```python
from build123d import *

# Parameters (mm, degrees)
EXTRUDE1_DEPTH = 12.7
EXTRUDE2_DEPTH = 216.9
SKETCH8_R      = 9.07761974
EXTRUDE3_DEPTH = 216.9


with BuildPart() as part:
    # Sketch1 → Extrude1 (new body)
    with BuildSketch(Plane(origin=(0, 0, 0), x_dir=(1, 0, 0), z_dir=(0, 1, 0))):
        with BuildLine():
            Line((-131.982271537, 76.2), (-21.997045256, 12.7))
            ThreePointArc((-21.997045256, 12.7), (0, 25.4), (21.997045256, 12.7))
            Line((21.997045256, 12.7), (131.982271537, 76.2))
            ThreePointArc((131.982271537, 76.2), (0, -152.4), (-131.982271537, 76.2))
        make_face()
    extrude(amount=EXTRUDE1_DEPTH)

    # Sketch2 → Extrude2 (cut, through all)
    with BuildSketch(Plane(origin=(0, 12.7, 0), x_dir=(1, 0, 0), z_dir=(0, 1, 0))):
        with BuildLine():
            Line((-122.312523376, 34.185473895), (-25.376324988, -1.096416941))
            ThreePointArc((-25.376324988, -1.096416941), (-20.043874739, -15.601380882), (-7.29146874, -24.33093676))
            Line((-7.29146874, -24.33093676), (-24.958114169, -124.523461794))
            ThreePointArc((-24.958114169, -124.523461794), (-108.255677623, -66.405634267), (-122.312523376, 34.185473895))
        make_face()
        with BuildLine():
            Line((25.376324988, -1.096416941), (122.312523376, 34.185473895))
            ThreePointArc((122.312523376, 34.185473895), (108.43851372, -66.106646732), (25.644983679, -124.38382054))
            Line((25.644983679, -124.38382054), (7.965532589, -24.118670995))
            ThreePointArc((7.965532589, -24.118670995), (20.258971151, -15.321034165), (25.376324988, -1.096416941))
        make_face()
    extrude(amount=-EXTRUDE2_DEPTH, mode=Mode.SUBTRACT)

    # Sketch8 → Extrude3 (cut, through all)
    with BuildSketch(Plane.XZ):
        with Locations(Location((0, 0, 0), (0, 0, 270))):
            Circle(SKETCH8_R)
    extrude(amount=-EXTRUDE3_DEPTH, mode=Mode.SUBTRACT)


solid = part.part
```
The model under review builds one solid part; all positions refer to its coordinate system, in mm. A direction names the side the tool comes from. Coordinates: 2 decimals unless noted, no trailing zeros. Order: outer loops, then holes, each group sorted by start corner. A loop starts at its lowest first (then second) coordinate and runs counter-clockwise, first axis right, second up. Notation, with made-up numbers: M 86,30.5 L 130,30.5 A17 cw 130,59.5 Z; hole C 42.25,12 d10. An arc over 180 degrees is marked long. One line per question, with ' | ' between items.
(1) Add section A-A, the plane x = 0. Write out the cut boundary in (y, z).
Geometry results:
outline: M 0,-25.4 L 12.7,-25.4 L 12.7,-9.08 L 0,-9.08 Z; M 0,9.08 L 12.7,9.08 L 12.7,152.4 L 0,152.4 Z
(2) Insertion check: pin 1 (4 mm diameter, centred on x = 80.5, y = 2, fed in from +Z); pin 2 (6 mm diameter, centred on y = 5, z = -9, fed in from +X); pin 3 (10 mm diameter, centred on x = -110.5, z = -33.5, fed in from -Y); pin 4 (1 mm diameter, centred on x = 93.5, y = 11, fed in from +Z). Each pin has a flat end and moves straight along its axis. Give the tip position at first contact, or say it passes through.
Geometry results:
pin 1: stops at z = 130.63 | pin 2: stops at x = 152.28 | pin 3: stops at y = 0 | pin 4: stops at z = 120.73
(3) Add section B-B, the plane y = 9.25. Write out the cut boundary in (x, z).
Geometry results:
outline: M -131.98,-76.2 L -22,-12.7 A25.4 ccw 22,-12.7 L 131.98,-76.2 A152.4 ccw long Z; hole M -122.31,-34.19 L -25.38,1.1 A25.4 cw -7.29,24.33 L -24.96,124.52 A127 ccw Z; hole C 0,0 d18.16; hole M 7.97,24.12 A25.4 cw 25.38,1.1 L 122.31,-34.19 A127 ccw 25.64,124.38 Z
(4) The part is to be moulded in two halves that separate along X. For faces 1 (the face through (-107.484, 6.439, 67.648)), 2 (the face through (2, 0, 36)), 3 (the face through (4.468, 6.261, 152.334)), 4 (the face through (-5.524, 6.261, 7.204)), say which applies: +X half, -X half, draft (parallel to the pull), parting line (faces both ways), or undercut.
Geometry results:
face 1: undercut | face 2: draft | face 3: parting line | face 4: undercut
(5) Add section C-C, the plane x = 91.5. Write out the cut boundary in (y, z), then the cut area to 3 significant figures.
Geometry results:
outline: M 0,-52.83 L 12.7,-52.83 L 12.7,-22.97 L 0,-22.97 Z; M 0,88.07 L 12.7,88.07 L 12.7,121.87 L 0,121.87 Z | area: 808 mm²
(6) Machinability: for faces 5 (the face through (-77.76, 6.261, -44.894)), 6 (the face through (20.13, 6.44, 15.49)), 7 (the face through (2, 12.7, 36)), which of the approach directions +Z, -Z, +X, -X, +Y, -Y give a long, thin tool a straight path to every point of the face, cutting with its end or side? Answer none if there is none.
Geometry results:
face 5: -Z, +Y, -Y | face 6: +Y, -Y | face 7: +Z, -Z, +X, -X, +Y
(7) For probe 1 along X at (y, z) = (9.75, 53); probe 2 along X at (y, z) = (4.25, 71); probe 3 along X at (y, z) = (4.75, -52), list the stretches that pass through material, from the lowest coordinate up. Write a range as from..to.
Geometry results:
probe 1: x = -142.89..-115.41, -12.35..13.06, 115.41..142.89 | probe 2: x = -134.85..-105.3, -15.52..16.23, 105.3..134.85 | probe 3: x = -143.25..-90.07, 90.07..143.25
